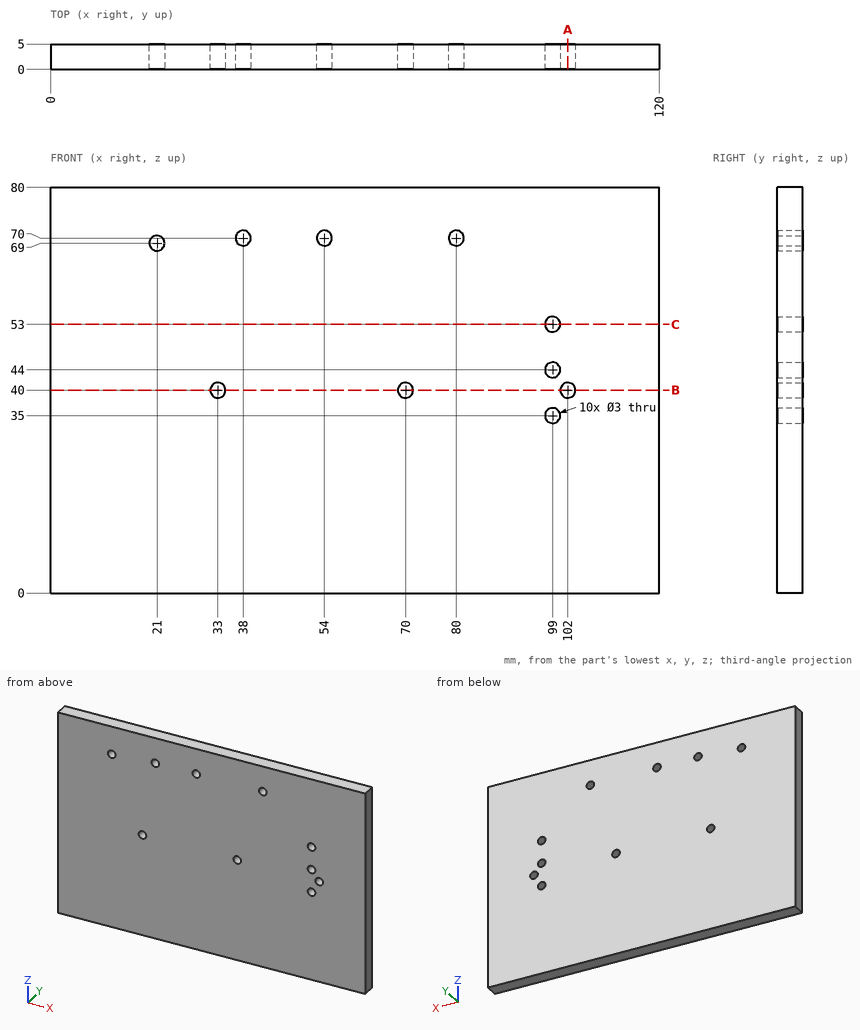
Drawing for the job (mm, zero at the part's lowest x, y, z). Round coordinates to 2 decimals unless told otherwise and drop trailing zeros. Loops run counter-clockwise (first coordinate to the right, second up) from the corner with the lowest first, then second, coordinate; pieces in that order, holes last. Notation, with made-up numbers: (64.25, -14) - (111.25, -14) arc R16 cw to (111.25, 6) - close; hole circle Ø1 at (68, -22.5). An arc over 180 degrees is marked (long way). Return JSON: item names as keys, results as strings. Group by question number.
Q1. Drill centre lines: line 1 along Z through (x, y) = (33, 1.3); line 2 along Z through (x, y) = (99.5, 2.1); line 3 along X through (y, z) = (3.75, 70). Where is each one in solid material? Low to high. Write a range as [from, to].
Q2. Band-saw the part on B-B on z = 40. Give the cut face in (x, y), plus the area to 3 significant figures.
Q3. Flat gauge pins, fed straight in: pin 1 Ø2.5 at (x, z) = (99, 35) entering from +Y; pin 2 Ø4 at (x, z) = (102, 40) entering from -Y. Where does each tip first touch, or does it go through?
Q4. Band-saw the part on A-A on x = 102. Give the cut face in (y, z).
Q5. Band-saw the part on C-C on z = 53. Give the cut face in (x, y), plus the area to 3 significant figures.
Solutions:
{
 "1": {"line 1": "z = [0, 38.5], [41.5, 80]", "line 2": "z = [0, 33.59], [36.41, 42.59], [45.41, 51.59], [54.41, 80]", "line 3": "x = [0, 19.88], [22.12, 36.5], [39.5, 52.5], [55.5, 78.5], [81.5, 120]"},
 "2": {"outline": "(0, 0) - (31.5, 0) - (31.5, 5) - (0, 5) - close; (34.5, 0) - (68.5, 0) - (68.5, 5) - (34.5, 5) - close; (71.5, 0) - (100.5, 0) - (100.5, 5) - (71.5, 5) - close; (103.5, 0) - (120, 0) - (120, 5) - (103.5, 5) - close", "area": "555 mm^2"},
 "3": {"pin 1": "passes through", "pin 2": "stops at y = 0"},
 "4": {"outline": "(0, 0) - (5, 0) - (5, 38.5) - (0, 38.5) - close; (0, 41.5) - (5, 41.5) - (5, 80) - (0, 80) - close"},
 "5": {"outline": "(0, 0) - (97.5, 0) - (97.5, 5) - (0, 5) - close; (100.5, 0) - (120, 0) - (120, 5) - (100.5, 5) - close", "area": "585 mm^2"}
}
